Input: part model. Units: mm. Frame: model coordinates. A direction names the side the tool comes from. Round coordinates to 2 decimals unless told otherwise and drop trailing zeros. Write each loop counter-clockwise with the first axis right and the second up, starting at its lowest first coordinate (ties: lowest second). Pieces come first, ordered by that corner, then holes. Notation, with made-up numbers: (-2.5, 31.25) -> (20.5, 31.25) arc R22 cw to (20.5, 65.25) -> close; hole circle Ø8 at (21, 12). An arc over 180 degrees is marked (long way). Use CSV: the item, a comma, the result in double quotes.
Autodesk Inventor part; units mm, degrees
ref_plane "YZ Plane" through (0, 0, 0) normal (1, 0, 0) x (0, 1, 0)
ref_plane "XZ Plane" through (0, 0, 0) normal (0, 1, 0) x (-1, 0, 0)
ref_plane "XY Plane" through (0, 0, 0) normal (0, 0, 1) x (1, 0, 0)
sketch "Sketch1" plane through (0, 0, 0) normal (0, 1, 0) x (-1, 0, 0)
  line L0 (0, 0) -> (-25.4, 0)
  line L1 (-25.4, 0) -> (-25.4, 76.2)
  line L2 (-25.4, 76.2) -> (0, 76.2)
  line L3 (0, 76.2) -> (0, 0)
  line L4 (-25.4, 76.2) -> (-76.2, 76.2)
  line L5 (-76.2, 76.2) -> (-76.2, 50.8)
  line L6 (-76.2, 50.8) -> (-25.4, 50.8)
  line L7 (-25.4, 50.8) -> (-25.4, 76.2)
  circle A0 centre (-63.5, 63.5) radius 2.5797
  circle A1 centre (-38.1, 63.5) radius 2.5797
  circle A2 centre (-12.7, 63.5) radius 2.5797
  circle A3 centre (-12.7, 38.1) radius 2.5797
  circle A4 centre (-12.7, 12.7) radius 2.5797
  dimension "d0" = 0
  dimension "d1" = 25.4
  dimension "d2" = 76.2
  dimension "d3" = 50.8
  dimension "d4" = 25.4
  dimension "d5" = 12.7
  dimension "d6" = 12.7
  dimension "d7" = 12.7
  dimension "d8" = 12.7
  dimension "d9" = 25.4
  dimension "d10" = 25.4
  dimension "d11" = 5.1594
  dimension "d12" = 5.1594
  dimension "d13" = 5.1594
  dimension "d14" = 5.1594
  dimension "d15" = 5.1594
  dimension "d16" = 12.7
  dimension "d17" = 12.7
  dimension "d18" = 12.7
  dimension "d19" = 25.4
  dimension "d20" = 12.7
extrude "Extrusion1" add sketch "Sketch1" along normal blind 2.54
equation "\"d6\" = d5"
equation "\"d7\" = d5"
equation "\"d12\" = d11"
equation "\"d13\" = d11"
equation "\"d14\" = d11"
equation "\"d15\" = d11"
properties part number "Bracing 3x3"
Item 1: First-contact query: pin 1 Ø1 at (x, y) = (12, 2) entering from -Z; pin 2 Ø4.5 at (x, z) = (12.7, 38.1) entering from -Y. Flat tips, straight axial feed; report the tip coordinate or a pass-through.
Worked answers:
pin 1,"stops at z = 0"
pin 2,"passes through"
Item 2: Pull-direction query (X, two-part tool) for faces 1 (the face through (13, 1, 0)), 2 (the face through (63.836, 1.252, 60.942)), 3 (the face through (76.2, 1, 64)); classes: +X half, -X half, draft (parallel to the pull), parting line (faces both ways), or undercut.
Worked answers:
face 1,"draft"
face 2,"undercut"
face 3,"+X half"
Item 3: Section query D-D on x = 38.1. Return the cut outline in (y, z), plus the area to 3 significant figures.
Worked answers:
outline,"(0, 50.8) -> (2.54, 50.8) -> (2.54, 60.92) -> (0, 60.92) -> close; (0, 66.08) -> (2.54, 66.08) -> (2.54, 76.2) -> (0, 76.2) -> close"
area,"51.4 mm²"
Item 4: Section query B-B on x = 12.7. Return the cut outline in (y, z), plus the area to 3 significant figures.
Worked answers:
outline,"(0, 0) -> (2.54, 0) -> (2.54, 10.12) -> (0, 10.12) -> close; (0, 15.28) -> (2.54, 15.28) -> (2.54, 35.52) -> (0, 35.52) -> close; (0, 40.68) -> (2.54, 40.68) -> (2.54, 60.92) -> (0, 60.92) -> close; (0, 66.08) -> (2.54, 66.08) -> (2.54, 76.2) -> (0, 76.2) -> close"
area,"154 mm²"
Item 5: Section query A-A on z = 38.1. Return the cut outline in (x, y).
Worked answers:
outline,"(0, 0) -> (10.12, 0) -> (10.12, 2.54) -> (0, 2.54) -> close; (15.28, 0) -> (25.4, 0) -> (25.4, 2.54) -> (15.28, 2.54) -> close"
Item 6: Line query: line 1 (Z direction, x = 12.7, y = 1.5); line 2 (X direction, y = 1.2, z = 38); line 3 (X direction, y = 1.3, z = 62). Output: solid intervals per line, ascending.
Worked answers:
line 1,"z = 0 to 10.12, 15.28 to 35.52, 40.68 to 60.92, 66.08 to 76.2"
line 2,"x = 0 to 10.12, 15.28 to 25.4"
line 3,"x = 0 to 10.6, 14.8 to 36, 40.2 to 61.4, 65.6 to 76.2"
Item 7: Set-up query: faces 4 (the face through (30, 0, 56)), 5 (the face through (25.4, 1, 25)). Return all of +Z, -Z, +X, -X, +Y, -Y with unobstructed straight access to the full face (end or side cutting, diameter ignored); none if empty.
Worked answers:
face 4,"+Z, -Z, +X, -X, -Y"
face 5,"-Z, +X, +Y, -Y"
Item 8: Section query C-C on z = 63.5. Return the cut outline in (x, y).
Worked answers:
outline,"(0, 0) -> (10.12, 0) -> (10.12, 2.54) -> (0, 2.54) -> close; (15.28, 0) -> (35.52, 0) -> (35.52, 2.54) -> (15.28, 2.54) -> close; (40.68, 0) -> (60.92, 0) -> (60.92, 2.54) -> (40.68, 2.54) -> close; (66.08, 0) -> (76.2, 0) -> (76.2, 2.54) -> (66.08, 2.54) -> close"
